Here's the drawing with two shaded views (mm, measured from the low corner). I have some questions. A direction names the side the tool comes from. Round coordinates to 2 decimals unless told otherwise and drop trailing zeros. Order: outer loops, then holes, each group sorted by start corner. A loop starts at its lowest first (then second) coordinate and runs counter-clockwise, first axis right, second up. Notation, with made-up numbers: (-9, 14.5) -> (44, 14.5) arc R16 ccw to (44, 28.5) -> close; hole circle Ø9 at (61.5, -37.5). An arc over 180 degrees is marked (long way). Answer in a Markdown table with one row per item.
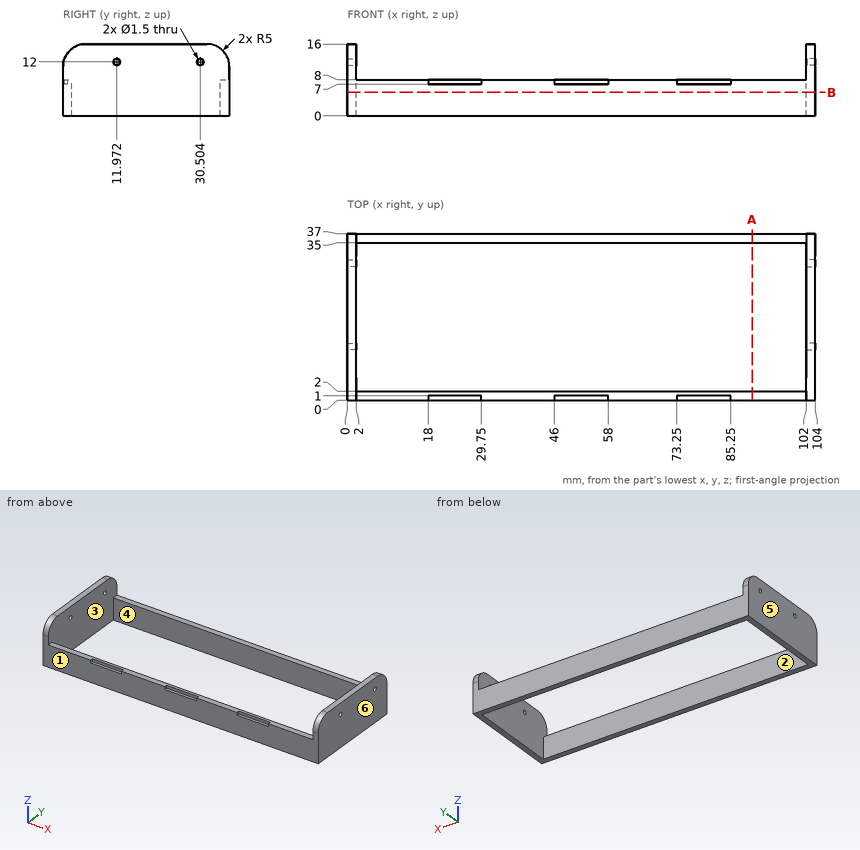
1. We'd pull the mould along X, two halves only. Please class the marked faces 3, 4, 5 and 6: released by +X, released by -X, zero draft, split by the parting line, or undercut.
Numbers:
| item | result |
|---|---|
| face 3 | undercut |
| face 4 | undercut |
| face 5 | released by -X |
| face 6 | released by +X |
2. Suppose I cut it at A-A on x = 90. Write out the boundary of the cut face in (y, z).
Numbers:
| item | result |
|---|---|
| outline | (0, 0) -> (2, 0) -> (2, 8) -> (0, 8) -> close; (35, 0) -> (37, 0) -> (37, 8) -> (35, 8) -> close |
3. Please list where these lines run through material, in increasing order: line 1 along Y through (x, z) = (87.5, 5.75); line 2 along X through (y, z) = (17, 3); line 3 along Y through (x, z) = (1.1, 12).
Numbers:
| item | result |
|---|---|
| line 1 | y = 0 to 2, 35 to 37 |
| line 2 | x = 0 to 2, 102 to 104 |
| line 3 | y = 0.1 to 11.22, 12.72 to 29.75, 31.25 to 36.9 |
4. For the marked faces 1 and 2, which set-ups out of +Z, -Z, +X, -X, +Y, -Y let a thin tool reach every point of the face, with its end or its side?
Numbers:
| item | result |
|---|---|
| face 1 | +Z, -Z, +X, -X, -Y |
| face 2 | +Z, -Z |
5. For pin 1 Ø0.5 at (x, z) = (78.5, 7.5) entering from -Y; pin 2 Ø1.4 at (y, z) = (11.97, 12) entering from -X; pin 3 Ø1.1 at (x, y) = (79, 0.5) entering from +Z, each with a flat end and sliding along its axis, tell me the tip position at first contact or that it passes through.
Numbers:
| item | result |
|---|---|
| pin 1 | stops at y = 1 |
| pin 2 | passes through |
| pin 3 | stops at z = 8 |
6. Suppose I cut it at B-B on z = 5.25. Write out the boundary of the cut face in (x, y), then the cut area to 3 significant figures.
Numbers:
| item | result |
|---|---|
| outline | (0, 0) -> (104, 0) -> (104, 37) -> (0, 37) -> close; hole (2, 2) -> (102, 2) -> (102, 35) -> (2, 35) -> close |
| area | 548 mm2 |
